Input: part model. Units: mm. Frame: model coordinates. Round coordinates to 2 decimals unless told otherwise and drop trailing zeros. Loops run counter-clockwise (first coordinate to the right, second up) from the corner with the lowest first, then second, coordinate; pieces in that order, holes last.
1) First-contact query: pin 1 (1 mm diameter, centred on x = 40, y = -52, fed in from -Z); pin 2 (4 mm diameter, centred on y = -67.5, z = 50, fed in from -X). Flat tips, straight axial feed; report the tip coordinate or a pass-through.
2) Section A-A, the plane z = 49.5. Return loops of the section in (x, y), and give its area (3 significant figures).
3) Ray query, line 1 along Y through (x, z) = (-147, 18.5); line 2 along X through (y, z) = (-73, 54); line 3 along Y through (x, z) = (-10, 53). Return the intervals inside material, ascending.
from build123d import *

# Parameters (mm, degrees)
CROQUIS1_W              = 520
CROQUIS1_H              = 330
SALIENTE_EXTRUIR1_DEPTH = 9
CROQUIS2_W              = 330
CROQUIS2_H              = 520
SALIENTE_EXTRUIR2_DEPTH = 50
REDONDEO1_R             = 20


with BuildPart() as part:
    # Croquis1 → Saliente-Extruir1 (new body)
    with BuildSketch(Plane(origin=(0, 0, 0), x_dir=(0, 1, 0), z_dir=(0, 0, 1))):
        Rectangle(CROQUIS1_W, CROQUIS1_H)
    extrude(amount=SALIENTE_EXTRUIR1_DEPTH)

    # Croquis2 → Saliente-Extruir2 (add)
    with BuildSketch(Plane.XY.offset(9)):
        Rectangle(CROQUIS2_W, CROQUIS2_H)
    extrude(amount=SALIENTE_EXTRUIR2_DEPTH)

    # Redondeo1
    redondeo1_edges = [part.edges().sort_by_distance(p)[0] for p in [
        (165, 0, 59),
        (0, 260, 59),
        (-165, 0, 59),
        (0, -260, 59),
        (165, 260, 29.5),
        (165, -260, 29.5),
        (-165, -260, 29.5),
        (-165, 260, 29.5),
    ]]
    fillet(redondeo1_edges, radius=REDONDEO1_R)


solid = part.part
Final values:
1. pin 1: stops at z = 0
1. pin 2: stops at x = -162.86
2. outline: (-162.02, -240) arc R17.02 ccw to (-145, -257.02) - (145, -257.02) arc R17.02 ccw to (162.02, -240) - (162.02, 240) arc R17.02 ccw to (145, 257.02) - (-145, 257.02) arc R17.02 ccw to (-162.02, 240) - close
2. area: 166,000 mm2
3. line 1: y = -259.9 to 259.9
3. line 2: x = -158.23 to 158.23
3. line 3: y = -254.28 to 254.28
